```python
from build123d import *

# Parameters (mm, degrees)
SKETCH_1_R          = 18
EXTRUDE_1_DEPTH     = 12
SKETCH_3_R          = 2.15
SKETCH_3_R_2        = 2.2
CUT_EXTRUDE_1_DEPTH = 29.142494559
SKETCH_4_R          = 5
CUT_EXTRUDE_2_DEPTH = 29.142494559


with BuildPart() as part:
    # 草图1 → 凸台-拉伸1 (new body)
    with BuildSketch(Plane.XY):
        Circle(SKETCH_1_R)
    extrude(amount=EXTRUDE_1_DEPTH)

    # 草图3 → 切除-拉伸1 (cut, through all)
    with BuildSketch(Plane.XY.offset(12)):
        with Locations((0, 9.715)):
            Circle(SKETCH_3_R)
        with Locations((8.413436798, -4.8575)):
            Circle(SKETCH_3_R)
        with Locations((-8.413436798, -4.8575)):
            Circle(SKETCH_3_R)
        with Locations((9.959292144, 5.75)):
            Circle(SKETCH_3_R_2)
        with Locations((0, -11.5)):
            Circle(SKETCH_3_R_2)
        with Locations((-9.959292144, 5.75)):
            Circle(SKETCH_3_R_2)
    extrude(amount=-CUT_EXTRUDE_1_DEPTH, mode=Mode.SUBTRACT)

    # 草图4 → 切除-拉伸2 (cut, through all)
    with BuildSketch(Plane.XY.offset(12)):
        Circle(SKETCH_4_R)
    extrude(amount=-CUT_EXTRUDE_2_DEPTH, mode=Mode.SUBTRACT)


solid = part.part
```
Read the model definition and answer for the solid it produces. Units are mm, in the model's axes. Give positions to 0.01 mm unless a question says otherwise; leave off trailing zeros. Order: outer loops, then holes, each group sorted by start corner. A loop starts at its lowest first (then second) coordinate and runs counter-clockwise, first axis right, second up.
(1) Find section B-B (y = 0). Give the vertices of the cut face in (x, z), plus the area to 3 significant figures.
(2) Given pin 1 (6 mm diameter, centred on x = 8, z = 3, fed in from -Y); pin 2 (2 mm diameter, centred on y = 2.5, z = 2.5, fed in from +X); pin 3 (2.5 mm diameter, centred on x = 0, y = -11.5, fed in from +Z); pin 4 (1 mm diameter, centred on x = 5, z = 3.5, fed in from -Y), each flat-ended and moving along its own axis, determine where each tip first touches the part or whether it passes through.
(3) Find section D-D (z = 9). Give the number of separate pieces and of enclosed holes in the cut face, plus the area to 3 significant figures.
(4) Straight lines are drawn through the part: L1, parallel to Y at x = 0, z = 9 (3 decimals); L2, parallel to Y at x = -10, z = 2; L3, parallel to X at y = -5.5, z = 4.75. For each, find the intervals that lie inside material, in ascending order.
(5) Find section C-C (x = -8.5). Give the vertices of the cut face in (y, z).
(6) Find section A-A (x = 0). Give the vertices of the cut face in (y, z) (3 decimals).
(7) For a pull along X with two mould halves and no side action, classify faces 1 (the flat face through (4, -4, 0)), 2 (the cylindrical face through (-2.343, 17.847, 5.916)), 3 (the cylindrical face through (-1.08, -4.88, 6.08)) as released by +X, released by -X, zero draft, split by the parting line, or undercut.
Result sheet:
1. outline: (-18, 0) - (-5, 0) - (-5, 12) - (-18, 12) - close; (5, 0) - (18, 0) - (18, 12) - (5, 12) - close
1. area: 312 mm2
2. pin 1: stops at y = -17.29
2. pin 2: stops at x = 17.94
2. pin 3: passes through
2. pin 4: stops at y = -17.43
3. separate pieces: 1
3. enclosed holes: 7
3. area: 850 mm2
4. L1: y = -18 to -13.7, -9.3 to -5, 5 to 7.565, 11.865 to 18
4. L2: y = -14.97 to -6.31, -3.41 to 3.55, 7.95 to 14.97
4. L3: x = -17.14 to -10.47, -6.36 to 6.36, 10.47 to 17.14
5. outline: (-15.87, 0) - (-7.01, 0) - (-7.01, 12) - (-15.87, 12) - close; (-2.71, 0) - (4.1, 0) - (4.1, 12) - (-2.71, 12) - close; (7.4, 0) - (15.87, 0) - (15.87, 12) - (7.4, 12) - close
6. outline: (-18, 0) - (-13.7, 0) - (-13.7, 12) - (-18, 12) - close; (-9.3, 0) - (-5, 0) - (-5, 12) - (-9.3, 12) - close; (5, 0) - (7.565, 0) - (7.565, 12) - (5, 12) - close; (11.865, 0) - (18, 0) - (18, 12) - (11.865, 12) - close
7. face 1: zero draft
7. face 2: split by the parting line
7. face 3: undercut
